from build123d import *

# Parameters (mm, degrees)
BASPROSKE_W         = 10
BASPROSKE_H         = 17
TOOTHCUT_DEPTH      = 27.038433133
TEETHCUTS_COUNT     = 15
BORSKE_R            = 10.5
BORE_DEPTH          = 10
SKETCH1_R           = 10.5
SKETCH1_R_2         = 1
SKETCH1_R_3         = 4.5
BOSS_EXTRUDE1_DEPTH = 5


with BuildPart() as part:
    # BasProSke → Base-Revolve (revolve)
    with BuildSketch(Plane(origin=(0, 0, 0), x_dir=(1, 0, 0), z_dir=(0, 1, 0)), mode=Mode.PRIVATE) as base_revolve_sk:
        with Locations((5, 8.5)):
            Rectangle(BASPROSKE_W, BASPROSKE_H)
    revolve(base_revolve_sk.sketch.rotate(Axis((-10, 0, 0), (1, 0, 0)), 180), axis=Axis((-10, 0, 0), (1, 0, 0)))

    # TooCutSke → ToothCut (cut, through all)
    with BuildSketch(Plane(origin=(0, 0, 0), x_dir=(0, 0, -1), z_dir=(1, 0, 0))):
        with BuildLine():
            ThreePointArc((1.050056448, 12.454813626), (0, 12.499), (-1.050056448, 12.454813626))
            ThreePointArc((-1.050056448, 12.454813626), (-1.638118106, 14.809604533), (-3.110934279, 16.73876737))
            ThreePointArc((-3.110934279, 16.73876737), (0, 17.0254), (3.110934279, 16.73876737))
            ThreePointArc((3.110934279, 16.73876737), (1.638118106, 14.809604533), (1.050056448, 12.454813626))
        make_face()
    toothcut = extrude(amount=TOOTHCUT_DEPTH, mode=Mode.SUBTRACT)

    # TeethCuts: ToothCut ×15 about axis
    teethcuts_axis = Axis((0, 0, 0), (1, 0, 0))
    for i in range(1, TEETHCUTS_COUNT):
        add(toothcut.rotate(teethcuts_axis, i * 360 / TEETHCUTS_COUNT), mode=Mode.SUBTRACT)

    # BorSke → Bore (cut, symmetric)
    with BuildSketch(Plane(origin=(0, 0, 0), x_dir=(0, 0, -1), z_dir=(1, 0, 0))):
        with Locations(Location((0, 0, 0), (0, 0, 180))):
            Circle(BORSKE_R)
    extrude(amount=BORE_DEPTH, both=True, mode=Mode.SUBTRACT)

    # Sketch1 → Boss-Extrude1 (add)
    with BuildSketch(Plane(origin=(0, 0, 0), x_dir=(0, 0, -1), z_dir=(1, 0, 0))):
        with Locations(Location((0, 0, 0), (0, 0, 180))):
            Circle(SKETCH1_R)
        with Locations((7, 0)):
            Circle(SKETCH1_R_2, mode=Mode.SUBTRACT)
        with Locations((-7, 0)):
            Circle(SKETCH1_R_2, mode=Mode.SUBTRACT)
        with Locations((0, 7)):
            Circle(SKETCH1_R_2, mode=Mode.SUBTRACT)
        with Locations((0, -7)):
            Circle(SKETCH1_R_2, mode=Mode.SUBTRACT)
        Circle(SKETCH1_R_3, mode=Mode.SUBTRACT)
    extrude(amount=BOSS_EXTRUDE1_DEPTH)


solid = part.part
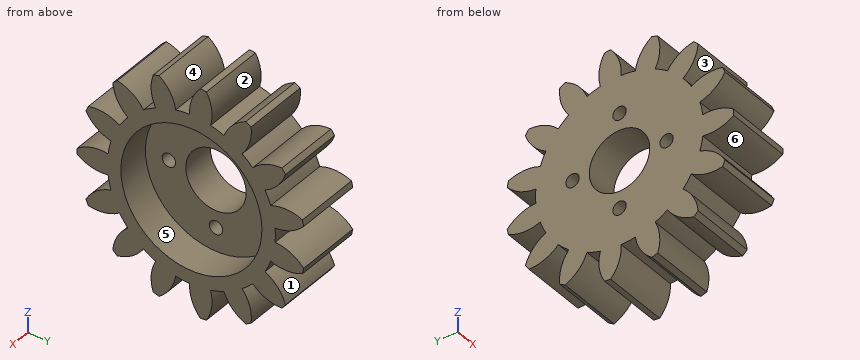
Could you check a few things on this model? Use its own coordinates, in mm. Face numbers are marked on the shaded views. A direction names the side the tool comes from. Give positions to 0.01 mm unless a question says otherwise; leave off trailing zeros. Order: outer loops, then holes, each group sorted by start corner. A loop starts at its lowest first (then second) coordinate and runs counter-clockwise, first axis right, second up.
Item 1: I'm going to push flat-ended pins straight in: pin 1 (2.5 mm diameter, centred on y = 0, z = 7, fed in from +X); pin 2 (6 mm diameter, centred on x = 7, z = -13, fed in from -Y); pin 3 (3 mm diameter, centred on x = 1.5, z = -3.5, fed in from -Y). Where does each tip first touch, or does it pass through?
Item 2: If we section it at D-D, the plane x = 3.25: Count the separate pieces of the cut face and the enclosed holes in it, plus the area to 3 significant figures.
Item 3: If we section it at B-B, the plane y = -14.5: Write out the boundary of the cut face in (x, z).
Item 4: If we section it at C-C, the plane y = 7: Write out the boundary of the cut face in (x, z).
Item 5: If we section it at A-A, the plane z = 0: Write out the boundary of the cut face in (x, y), plus the area to 3 significant figures.
Item 6: If we mould it in two halves opening along Y, with no side actions, what happens to the marked faces 1, 2 and 3? For each: pulls with the +Y half, pulls with the -Y half, needs draft (parallel to the pull), parting line crosses it, or undercut.
Item 7: I need wall thicknesses on line 1 (Y direction, x = 2.8, z = 0); line 2 (Y direction, x = 4, z = 13); line 3 (Y direction, x = 1.4, z = 7). Which ranges of each line are inside material? Lowest first, please.
Item 8: For the marked faces 4, 5 and 6, which set-ups out of +Z, -Z, +X, -X, +Y, -Y let a thin tool reach every point of the face, with its end or its side?
Values:
1. pin 1: stops at x = 5
1. pin 2: stops at y = -11.71
1. pin 3: stops at y = -14.52
2. separate pieces: 1
2. enclosed holes: 5
2. area: 597 mm2
3. outline: (0, -7.46) - (10, -7.46) - (10, -4.98) - (0, -4.98) - close; (0, -1.55) - (10, -1.55) - (10, 1.55) - (0, 1.55) - close; (0, 4.98) - (10, 4.98) - (10, 7.46) - (0, 7.46) - close
4. outline: (0, -14.33) - (10, -14.33) - (10, -7.83) - (5, -7.83) - (5, -1) - (0, -1) - close; (0, 1) - (5, 1) - (5, 7.83) - (10, 7.83) - (10, 14.33) - (0, 14.33) - close
5. outline: (0, -17) - (10, -17) - (10, -10.5) - (5, -10.5) - (5, -8) - (0, -8) - close; (0, -6) - (5, -6) - (5, -4.5) - (0, -4.5) - close; (0, 4.5) - (5, 4.5) - (5, 6) - (0, 6) - close; (0, 8) - (5, 8) - (5, 10.5) - (10, 10.5) - (10, 12.5) - (0, 12.5) - close
5. area: 125 mm2
6. face 1: pulls with the +Y half
6. face 2: undercut
6. face 3: pulls with the -Y half
7. line 1: y = -17 to -8, -6 to -4.5, 4.5 to 6, 8 to 12.5
7. line 2: y = -5.9 to -2.5, -0.27 to 3.02, 5.65 to 8.88
7. line 3: y = -15.49 to -11.67, -10.35 to -1, 1 to 12.37
8. face 4: +Z, +X, -X
8. face 5: +X
8. face 6: +X, -X
